```python
from build123d import *

# Parameters (mm, degrees)
SKIZZE1_W                       = 35
SKIZZE1_H                       = 75
AUFSATZ_LINEAR_AUSTRAGEN1_DEPTH = 1.5
SKIZZE2_W                       = 11.63
SKIZZE2_H                       = 5
SKIZZE2_W_2                     = 11.62
SKIZZE2_W_3                     = 1.75
SCHNITT_LINEAR_AUSTRAGEN1_DEPTH = 1.5
SCHNITT_LINEAR_AUSTRAGEN3_DEPTH = 1.5


with BuildPart() as part:
    # Skizze1 → Aufsatz-Linear austragen1 (new body)
    with BuildSketch(Plane.XY):
        with Locations((17.5, 37.5)):
            Rectangle(SKIZZE1_W, SKIZZE1_H)
    extrude(amount=AUFSATZ_LINEAR_AUSTRAGEN1_DEPTH)

    # Skizze2 → Schnitt-Linear austragen1 (cut)
    with BuildSketch(Plane.XY.offset(1.5)):
        with Locations((5.815, 2.5)):
            Rectangle(SKIZZE2_W, SKIZZE2_H)
        with Locations((29.19, 2.5)):
            Rectangle(SKIZZE2_W_2, SKIZZE2_H)
        with Locations((17.505, 2.5)):
            Rectangle(SKIZZE2_W_3, SKIZZE2_H)
    extrude(amount=-SCHNITT_LINEAR_AUSTRAGEN1_DEPTH, mode=Mode.SUBTRACT)

    # Skizze6 → Schnitt-Linear austragen3 (cut)
    with BuildSketch(Plane.XY.offset(1.5)):
        Polygon((8.694210646, 55.87711337), (17.317097276, 64.5), (18.831310838, 64.5), (18.831310838, 17), (17.831310838, 17), (17.831310838, 63.5), (17.731310838, 63.5), (10.108424208, 55.87711337), align=None)
    extrude(amount=-SCHNITT_LINEAR_AUSTRAGEN3_DEPTH, mode=Mode.SUBTRACT)


solid = part.part
```
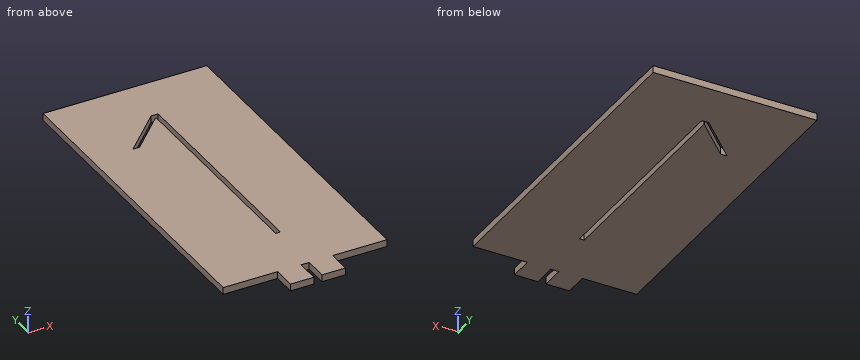
Work out the finished part from the listing and answer in its coordinate system (mm). Round coordinates to 2 decimals unless told otherwise and drop trailing zeros. Write each loop counter-clockwise with the first axis right and the second up, starting at its lowest first coordinate (ties: lowest second). Pieces come first, ordered by that corner, then holes.
1) A cutting plane is placed at D-D on x = 26. Determine the outline of the cut face in (y, z), and give its area (3 significant figures).
2) A cutting plane is placed at B-B on z = 0.25. Determine the outline of the cut face in (x, y), and give its area (3 significant figures).
3) A cutting plane is placed at C-C on x = 14. Determine the outline of the cut face in (y, z), and give its area (3 significant figures).
4) Consider probe 1 along X at (y, z) = (48.5, 1); probe 2 along Y at (x, z) = (7, 0.75); probe 3 along Y at (x, z) = (17, 0.3). Determine where each line is inside the solid, lowest interval first.
5) Flat-ended cylindrical pins translate along their axes: P1, Ø0.8, axis at y = 3.5, z = 1, coming from the -X side; P2, Ø0.8, axis at x = 5.5, z = 0.5, coming from the -Y side. Find the tip coordinate at first contact, or state that the pin passes through.
6) A cutting plane is placed at A-A on y = 23. Determine the outline of the cut face in (x, z).
Entries:
1. outline: (5, 0) - (75, 0) - (75, 1.5) - (5, 1.5) - close
1. area: 105 mm2
2. outline: (0, 5) - (11.63, 5) - (11.63, 0) - (16.63, 0) - (16.63, 5) - (18.38, 5) - (18.38, 0) - (23.38, 0) - (23.38, 5) - (35, 5) - (35, 75) - (0, 75) - close; hole (8.69, 55.88) - (10.11, 55.88) - (17.73, 63.5) - (17.83, 63.5) - (17.83, 17) - (18.83, 17) - (18.83, 64.5) - (17.32, 64.5) - close
2. area: 2,440 mm2
3. outline: (0, 0) - (59.77, 0) - (59.77, 1.5) - (0, 1.5) - close; (61.18, 0) - (75, 0) - (75, 1.5) - (61.18, 1.5) - close
3. area: 110 mm2
4. probe 1: x = 0 to 17.83, 18.83 to 35
4. probe 2: y = 5 to 75
4. probe 3: y = 5 to 62.77, 64.18 to 75
5. P1: stops at x = 11.63
5. P2: stops at y = 5
6. outline: (0, 0) - (17.83, 0) - (17.83, 1.5) - (0, 1.5) - close; (18.83, 0) - (35, 0) - (35, 1.5) - (18.83, 1.5) - close
